Verification items for the finished model (mm, model axes). A direction names the side the tool comes from. Round coordinates to 2 decimals unless told otherwise and drop trailing zeros. Write each loop counter-clockwise with the first axis right and the second up, starting at its lowest first coordinate (ties: lowest second). Pieces come first, ordered by that corner, then holes. Notation, with made-up numbers: M -1,47 L 7,47 A15 ccw 7,67 Z; hole C -5.5,6.5 d6. An arc over 180 degrees is marked long. One line per item, written item: value. Start each with the question number.
Item 1: Draft check along Y on faces 1 (the face through (472.283, -75.133, 15.867)), 2 (the face through (-7, 0, 1)), 3 (the face through (-395, -57.15, -39)), 4 (the face through (392, -95.25, -39)). Enter one of: +Y half, -Y half, draft (parallel to the pull), parting line (faces both ways), or undercut.
Item 2: Section check A-A, the plane x = 336.5. Record the cut outline in (y, z).
Item 3: Tool access check on faces 5 (the face through (-385, -76, 0)), 6 (the face through (392, -57.15, -39)), 7 (the face through (6, -75, 76.2)). Record the directions out of +Z, -Z, +X, -X, +Y, -Y that give a thin tool (end or side, any length) a straight path to the whole face; none if there is none.
Item 4: Gauge pin test, flat ends, axial feed: pin 1 (8 mm diameter, centred on y = -75, z = -57, fed in from +X); pin 2 (12 mm diameter, centred on y = -84, z = 53.5, fed in from +X) (3 decimals); pin 3 (19 mm diameter, centred on y = -74, z = -38, fed in from -X). Record the tip position at first contact, or that the pin passes through.
Item 5: Thickness scan on probe 1 along Y at (x, z) = (-451, -30.5); probe 2 along X at (y, z) = (-124.5, -60); probe 3 along X at (y, z) = (-81, 60). Record the ranges inside material, lowest first. Write a range as from..to.
Item 6: Section check D-D, the plane z = -47.5. Record the cut outline in (x, y) (3 decimals), then the cut area to 3 significant figures.
Item 7: Section check B-B, the plane y = -80. Record the cut outline in (x, z).
Item 8: Section check C-C, the plane z = 17. Record the cut outline in (x, y).
from build123d import *

# Parameters (mm, degrees)
F1_DEPTH = 152.4
F2_W     = 203.2
F2_H     = 38.1
F3_DEPTH = 76.2


with BuildPart() as f1:
    # F0 (on Front) → F1 (new body)
    with BuildSketch(Plane.XZ):
        Polygon((457.2, 76.2), (-457.2, 76.2), (-495.3, -76.2), (495.3, -76.2), align=None)
    extrude(amount=F1_DEPTH)

    # F2 (on face) → F3 (cut)
    with BuildSketch(Plane(origin=(0, 0, -76.2), x_dir=(1, 0, 0), z_dir=(0, 0, -1))):
        with Locations((-393.7, 76.2)):
            Rectangle(F2_W, F2_H)
        with Locations((393.7, 76.2)):
            Rectangle(F2_W, F2_H)
    extrude(amount=-F3_DEPTH, mode=Mode.SUBTRACT)


solid = f1.part
Response values:
1. face 1: draft
1. face 2: +Y half
1. face 3: undercut
1. face 4: undercut
2. outline: M -152.4,-76.2 L -95.25,-76.2 L -95.25,0 L -57.15,0 L -57.15,-76.2 L 0,-76.2 L 0,76.2 L -152.4,76.2 Z
3. face 5: -Z, -X
3. face 6: -Z, +X
3. face 7: +Z, +X, -X, +Y, -Y
4. pin 1: stops at x = 292.1
4. pin 2: stops at x = 464.375
4. pin 3: stops at x = -292.1
5. probe 1: y = -152.4..-95.25, -57.15..0
5. probe 2: x = -491.25..491.25
5. probe 3: x = -461.25..461.25
6. outline: M -488.125,-152.4 L 488.125,-152.4 L 488.125,-95.25 L 292.1,-95.25 L 292.1,-57.15 L 488.125,-57.15 L 488.125,0 L -488.125,0 L -488.125,-57.15 L -292.1,-57.15 L -292.1,-95.25 L -488.125,-95.25 Z
6. area: 134,000 mm2
7. outline: M -476.25,0 L -292.1,0 L -292.1,-76.2 L 292.1,-76.2 L 292.1,0 L 476.25,0 L 457.2,76.2 L -457.2,76.2 Z
8. outline: M -472,-152.4 L 472,-152.4 L 472,0 L -472,0 Z
